Input: part model. Units: mm. Frame: model coordinates. A direction names the side the tool comes from. Coordinates: 2 decimals unless noted, no trailing zeros. Loops run counter-clockwise (first coordinate to the right, second up) from the corner with the lowest first, then second, coordinate; pieces in that order, holes last.
(1) Section B-B, the plane y = 0. Return loops of the section in (x, z), then the cut area to 3 significant figures.
(2) Set-up query: faces 1 (the face through (0, 3, 175)), 2 (the face through (0, 3, 12)), 3 (the face through (0, 2, 6)), 4 (the face through (0, 2, 181)). Return all of +Z, -Z, +X, -X, +Y, -Y with unobstructed straight access to the full face (end or side cutting, diameter ignored); none if empty.
(3) Line query: L1, parallel to Z at x = 2.75, y = 2.5; L2, parallel to Y at x = -0.25, z = 142.5; L3, parallel to X at y = -0.5, z = 25. Output: solid intervals per line, ascending.
(4) Section C-C, the plane z = 149. Return loops of the section in (x, y), then the cut area to 3 significant figures.
(5) Contact query for flat-ended pins moving along their axis: P1, Ø2, axis at x = -2, z = 123, coming from the +Y side; P2, Ø2, axis at y = -1.5, z = 83.5, coming from the -X side; P3, Ø1.5, axis at y = 3, z = 151, coming from the +X side. Output: stop coordinate, or through.
(6) Section A-A, the plane x = 0. Return loops of the section in (y, z), then the cut area to 3 significant figures.
```python
from build123d import *

# Parameters (mm, degrees)
ESBO_O1_R                  = 6.35
RESSALTO_EXTRUS_O1_DEPTH   = 187
ESBO_O2_R                  = 12.7
ESBO_O2_R_2                = 4
CORTE_EXTRUS_O1_DEPTH      = 188.215504166
CORTE_EXTRUS_O2_DEPTH      = 188.085541932
CORTE_EXTRUS_O2_DEPTH_BACK = 188.085541932
ESBO_O3_W                  = 12
ESBO_O3_H                  = 10
ESBO_O5_W                  = 12
ESBO_O5_H                  = 10


with BuildPart() as part:
    # Esboço1 → Ressalto-extrusão1 (new body)
    with BuildSketch(Plane.XY):
        Circle(ESBO_O1_R)
    extrude(amount=RESSALTO_EXTRUS_O1_DEPTH)

    # Esboço2 → Corte-extrusão1 (cut, through all)
    with BuildSketch(Plane.XY.offset(187)):
        Circle(ESBO_O2_R)
        Circle(ESBO_O2_R_2, mode=Mode.SUBTRACT)
    extrude(amount=-CORTE_EXTRUS_O1_DEPTH, mode=Mode.SUBTRACT)

    # Esboço3 → Corte-extrusão2 (cut, two sides: drawn at the far end of the back side and taken through both)
    with BuildSketch(Plane(origin=(0, 0, 0), x_dir=(0, 0, -1), z_dir=(1, 0, 0)).offset(-CORTE_EXTRUS_O2_DEPTH_BACK)):
        with Locations((-181, 7)):
            Rectangle(ESBO_O3_W, ESBO_O3_H)
        with Locations((-6, 7)):
            Rectangle(ESBO_O3_W, ESBO_O3_H)
    extrude(amount=CORTE_EXTRUS_O2_DEPTH + CORTE_EXTRUS_O2_DEPTH_BACK, mode=Mode.SUBTRACT)

    # Esboço5 → Corte-Revolução2 (revolve, cut)
    with BuildSketch(Plane(origin=(0, 0, 0), x_dir=(0, 0, -1), z_dir=(1, 0, 0))):
        with Locations((-181, 8)):
            Rectangle(ESBO_O5_W, ESBO_O5_H)
        with Locations((-6, 8)):
            Rectangle(ESBO_O5_W, ESBO_O5_H)
    revolve(axis=Axis((0, 0, 0), (0, 0, 1)), mode=Mode.SUBTRACT)


solid = part.part
```
Report:
1. outline: (-4, 12) - (-3, 12) - (-3, 0) - (3, 0) - (3, 12) - (4, 12) - (4, 175) - (3, 175) - (3, 187) - (-3, 187) - (-3, 175) - (-4, 175) - close
1. area: 1,450 mm2
2. face 1: +Z
2. face 2: -Z
2. face 3: -Z, +X, -X, +Y
2. face 4: +Z, +X, -X, +Y
3. L1: z = 12 to 175
3. L2: y = -3.99 to 3.99
3. L3: x = -3.97 to 3.97
4. outline: circle Ø8 at (0, 0)
4. area: 50.3 mm2
5. P1: stops at y = 3.87
5. P2: stops at x = -3.97
5. P3: stops at x = 3.31
6. outline: (-4, 12) - (-3, 12) - (-3, 0) - (2, 0) - (2, 12) - (4, 12) - (4, 175) - (2, 175) - (2, 187) - (-3, 187) - (-3, 175) - (-4, 175) - close
6. area: 1,420 mm2
